The model under review builds one solid part; all positions refer to its coordinate system, in mm. A direction names the side the tool comes from. Give positions to 0.01 mm unless a question says otherwise; leave off trailing zeros. Order: outer loops, then holes, each group sorted by start corner. A loop starts at its lowest first (then second) coordinate and runs counter-clockwise, first axis right, second up.
```python
from build123d import *

# Parameters (mm, degrees)
SKETCH_1_W           = 145
SKETCH_1_H           = 100
EXTRUDE_1_DEPTH      = 1
SKETCH_2_W           = 55.047445891
SKETCH_2_H           = 29.312826224
EXTRUDE_2_DEPTH      = 4
SKETCH_3_R           = 1.75
SKETCH_3_R_2         = 1.682307007
CUT_EXTRUDE_1_DEPTH  = 89.211393822
EXTRUDE_3_DEPTH      = 5
EXTRUDE_3_DEPTH_BACK = 5
EXTRUDE_4_DEPTH      = 5
EXTRUDE_4_DEPTH_BACK = 5
FILLET_1_R           = 10
FILLET_3_R           = 10
FILLET_4_R           = 5
FILLET_5_R           = 10


with BuildPart() as part:
    # Эскиз1 → Бобышка-Вытянуть1 (new body)
    with BuildSketch(Plane(origin=(0, 0, 0), x_dir=(1, 0, 0), z_dir=(0, 1, 0))):
        Rectangle(SKETCH_1_W, SKETCH_1_H)
    extrude(amount=EXTRUDE_1_DEPTH)

    # Эскиз2 → Бобышка-Вытянуть2 (add)
    with BuildSketch(Plane(origin=(0, 1, 0), x_dir=(1, 0, 0), z_dir=(0, 1, 0))):
        with BuildLine():
            Line((70, -35), (70, 35))
            ThreePointArc((70, 35), (68.535533919, 38.535533893), (65.000000038, 40))
            Line((65.000000038, 40), (5, 40))
            Line((5, 40), (5, 50))
            Line((5, 50), (-5, 50))
            Line((-5, 50), (-5, 40))
            Line((-5, 40), (-65, 40))
            ThreePointArc((-65, 40), (-68.535533906, 38.535533906), (-70, 35))
            Line((-70, 35), (-70, -35))
            ThreePointArc((-70, -35), (-68.535533906, -38.535533906), (-65, -40))
            Line((-65, -40), (-5, -40))
            Line((-5, -40), (-5, -50))
            Line((-5, -50), (5, -50))
            Line((5, -50), (5, -40))
            Line((5, -40), (64.999999981, -40))
            ThreePointArc((64.999999981, -40), (68.535533899, -38.535533913), (70, -35))
        make_face()
        with Locations((-32.523722945, -19.656413112)):
            Rectangle(SKETCH_2_W, SKETCH_2_H, mode=Mode.SUBTRACT)
        with Locations((32.523722945, -19.656413112)):
            Rectangle(SKETCH_2_W, SKETCH_2_H, mode=Mode.SUBTRACT)
        with Locations((-32.523722945, 19.656413112)):
            Rectangle(SKETCH_2_W, SKETCH_2_H, mode=Mode.SUBTRACT)
        with Locations((32.523722945, 19.656413112)):
            Rectangle(SKETCH_2_W, SKETCH_2_H, mode=Mode.SUBTRACT)
    extrude(amount=EXTRUDE_2_DEPTH)

    # Эскиз3 → Вырез-Вытянуть1 (cut, through all)
    with BuildSketch(Plane(origin=(0, 5, 0), x_dir=(1, 0, 0), z_dir=(0, 1, 0))):
        with Locations(Location((-65, 35, 0), (0, 0, 270))):
            Circle(SKETCH_3_R)
        with Locations(Location((-65, -35, 0), (0, 0, 270))):
            Circle(SKETCH_3_R)
        with Locations(Location((65, -35, 0), (0, 0, 270))):
            Circle(SKETCH_3_R_2)
        with Locations(Location((65, 35, 0), (0, 0, 270))):
            Circle(SKETCH_3_R)
    extrude(amount=-CUT_EXTRUDE_1_DEPTH, mode=Mode.SUBTRACT)

    # Эскиз4 → Бобышка-Вытянуть3 (add, two sides: drawn at the far end of the back side and taken through both)
    with BuildSketch(Plane.XY.offset(-EXTRUDE_3_DEPTH_BACK)):
        Polygon((-72.5, 0), (-62.5, 0), (-63.077350269, 1), (-70, 1), (-70, 5), (-65.386751346, 5), (-79.820508076, 30), (-89.820508076, 30), align=None)
        Polygon((79.820508076, 30), (62.5, 0), (72.5, 0), (89.820508076, 30), align=None)
    extrude(amount=EXTRUDE_3_DEPTH + EXTRUDE_3_DEPTH_BACK)

    # Эскиз5 → Бобышка-Вытянуть4 (add, two sides: drawn at the far end of the back side and taken through both)
    with BuildSketch(Plane(origin=(0, 0, 0), x_dir=(0, 0, -1), z_dir=(1, 0, 0)).offset(-EXTRUDE_4_DEPTH_BACK)):
        Polygon((-50, 1), (-40.577350269, 1), (-57.320508076, 30), (-67.320508076, 30), (-50, 0), align=None)
        Polygon((50, 0), (40, 0), (57.320508076, 30), (67.320508076, 30), align=None)
    extrude(amount=EXTRUDE_4_DEPTH + EXTRUDE_4_DEPTH_BACK)

    # Скругление1
    fillet_1_edges = [part.edges().sort_by_distance(p)[0] for p in [
        (72.5, 0.5, 50),
        (-72.5, 0.5, 50),
        (-72.5, 0.5, -50),
        (72.5, 0.5, -50),
    ]]
    fillet(fillet_1_edges, radius=FILLET_1_R)

    # Скругление3
    fillet_3_edges = [part.edges().sort_by_distance(p)[0] for p in [
        (5, 3, -34.312826224),
        (60.047445891, 3, -34.312826224),
        (60.047445891, 3, 5),
        (60.047445891, 3, 34.312826224),
        (-5, 3, 5),
        (-60.047445891, 3, 5),
        (-5, 3, 34.312826224),
        (-60.047445891, 3, 34.312826224),
        (-60.047445891, 3, -5),
        (-60.047445891, 3, -34.312826224),
        (5, 3, -5),
        (60.047445891, 3, -5),
        (-5, 3, -34.312826224),
        (-5, 3, -5),
        (5, 3, 34.312826224),
        (5, 3, 5),
    ]]
    fillet(fillet_3_edges, radius=FILLET_3_R)

    # Скругление4
    fillet_4_edges = [part.edges().sort_by_distance(p)[0] for p in [
        (0, 5, 42.886751346),
        (-65.386751346, 5, 0),
        (65.386751346, 5, 0),
        (0, 5, -42.886751346),
    ]]
    fillet(fillet_4_edges, radius=FILLET_4_R)

    # Скругление5
    fillet_5_edges = [part.edges().sort_by_distance(p)[0] for p in [
        (-79.820508076, 30, 0),
        (79.820508076, 30, 0),
        (0, 30, 57.320508076),
        (0, 30, -57.320508076),
    ]]
    fillet(fillet_5_edges, radius=FILLET_5_R)


solid = part.part
```
Item 1: For line 1 (X direction, y = 2, z = -35); line 2 (Z direction, x = -65, y = 3); line 3 (X direction, y = 21.5, z = -60.5), list the stretches that pass through material, from the lowest coordinate up.
Values found:
line 1: x = -70 to -66.75, -63.25 to 63.25, 66.75 to 70
line 2: z = -40 to -36.75, -33.25 to 33.25, 36.75 to 40
line 3: x = -5 to 5
Item 2: Take a section at C-C (x = -12.5). Give the boundary of the cut face in (y, z), and give its area (3 significant figures).
Values found:
outline: (0, -50) - (1, -50) - (1, -40) - (5, -40) - (5, -34) - (1, -34) - (1, -5.32) - (5, -5.32) - (5, 5.32) - (1, 5.32) - (1, 34) - (5, 34) - (5, 40) - (1, 40) - (1, 50) - (0, 50) - close
area: 191 mm2
Item 3: Clearance check with flat-ended pins moving along their axes: pin 1 Ø23.5 at (x, z) = (39.5, -27) entering from +Y; pin 2 Ø2 at (x, y) = (25.5, 2.5) entering from -Z; pin 3 Ø3 at (x, y) = (39, 2) entering from -Z. State where each tip first meets the part, or that it passes through.
Values found:
pin 1: stops at y = 5
pin 2: stops at z = -40
pin 3: stops at z = -50
Item 4: Take a section at B-B (y = 20). Give the boundary of the cut face in (x, z), and give its area (3 significant figures).
Values found:
outline: (-84.05, -5) - (-74.05, -5) - (-74.05, 5) - (-84.05, 5) - close; (-5, -61.55) - (5, -61.55) - (5, -51.55) - (-5, -51.55) - close; (-5, 51.55) - (5, 51.55) - (5, 61.55) - (-5, 61.55) - close; (74.05, -5) - (84.05, -5) - (84.05, 5) - (74.05, 5) - close
area: 400 mm2
Item 5: Take a section at D-D (z = 47.5). Give the boundary of the cut face in (x, y).
Values found:
outline: (-69.11, 0) - (69.11, 0) - (69.11, 1) - (5, 1) - (5, 12.99) - (-5, 12.99) - (-5, 1) - (-69.11, 1) - close
Item 6: Take a section at A-A (z = 22.5). Give the boundary of the cut face in (x, y), and give its area (3 significant figures).
Values found:
outline: (-72.5, 0) - (72.5, 0) - (72.5, 1) - (70, 1) - (70, 5) - (60.05, 5) - (60.05, 1) - (5, 1) - (5, 5) - (-5, 5) - (-5, 1) - (-60.05, 1) - (-60.05, 5) - (-70, 5) - (-70, 1) - (-72.5, 1) - close
area: 265 mm2
Item 7: For faces 1 (the cylindrical face through (0.07, 5.652, -42.468)), 2 (the cylindrical face through (-57.2, 3.03, 8.01)), 3 (the flat face through (-81.28, 15.21, -0.07)), 4 (the cylindrical face through (-64.968, 5.652, 0.07)), 5 (the cylindrical face through (-69, 3, 38)), list the 3-axis set-ups (+Z, -Z, +X, -X, +Y, -Y) from which the entire face can be reached by the end or side of a thin tool; tool diameter is ignored.
Values found:
face 1: +X, -X, +Y
face 2: +Y
face 3: +Z, -Z, -X, -Y
face 4: +Z, -Z, +Y
face 5: +Z, -X, +Y
Item 8: Draft analysis for pull direction X (two halves, no side actions). For faces 6 (the flat face through (70, 3, -20)), 7 (the cylindrical face through (57.04, 3.03, -7.85)), 8 (the flat face through (41, 1, 42)), state which applies: released by +X, released by -X, zero draft, split by the parting line, or undercut.
Values found:
face 6: released by +X
face 7: undercut
face 8: zero draft
